Autodesk Inventor part; units mm, degrees
ref_plane "YZ Plane" through (0, 0, 0) normal (1, 0, 0) x (0, 1, 0)
ref_plane "XZ Plane" through (0, 0, 0) normal (0, 1, 0) x (-1, 0, 0)
ref_plane "XY Plane" through (0, 0, 0) normal (0, 0, 1) x (1, 0, 0)
sketch "Sketch1" plane through (0, 0, 0) normal (0, 1, 0) x (-1, 0, 0)
  circle A0 centre (30, -37.5) radius 2
  circle A1 centre (-30, -37.5) radius 2
  circle A2 centre (-30, 37.5) radius 2
  circle A3 centre (30, 37.5) radius 2
  arc A4 (27.9205, -42.0236) -> (32.0065, -32.9436) centre (30, -37.5) ccw
  line L0 (-8.045, -32.9204) -> (0.0364, -32.9204)
  line L1 (-8.045, -32.9204) -> (8.1178, -32.9204)
  line L2 (-8.0814, 33) -> (8.0814, 33)
  line L3 (27.9205, -42.0236) -> (8.1178, -32.9204)
  line L4 (32.0431, -32.9598) -> (8.1178, -22.3088)
  circle A5 centre (-30, -37.5) radius 2
  arc A6 (-31.9701, -32.864) -> (-27.8841, -41.944) centre (-29.9636, -37.4204) ccw
  line L5 (-27.9205, -41.9606) -> (-8.045, -32.9204)
  line L6 (-32.0067, -32.8802) -> (-8.045, -22.213)
  circle A7 centre (30, 37.5) radius 2
  circle A8 centre (-30, 37.5) radius 2
  arc A9 (32.0065, 32.9436) -> (27.9205, 42.0236) centre (30, 37.5) ccw
  line L7 (-8.0814, 33) -> (0, 33)
  line L8 (-8.0814, 33) -> (8.0814, 33)
  line L9 (27.9569, 42.0402) -> (8.0814, 33)
  line L10 (32.0278, 32.953) -> (8.1178, 22.341)
  line L11 (-27.9569, 42.0402) -> (-8.0814, 33)
  circle A10 centre (-30, 37.5) radius 2
  arc A11 (-27.9205, 42.0236) -> (-32.0065, 32.9436) centre (-30, 37.5) ccw
  line L12 (-32.0431, 32.9598) -> (-8.045, 22.2764)
  circle A12 centre (0, -22) radius 1.5
  circle A13 centre (0, 0) radius 1.5
  circle A14 centre (0, 22) radius 1.5
  line L13 (8.1178, 22.341) -> (8.1178, -22.3088)
  line L14 (-8.045, -22.213) -> (-8.045, 22.2764)
extrude "Extrusion1" add sketch "Sketch1" along normal blind 6
sketch "Sketch2" plane through (0, 6, 0) normal (0, 1, 0) x (1, 0, 0)
  circle A0 centre (-30, 37.5) radius 2
  circle A1 centre (-30, 37.5) radius 3.5
  circle A2 centre (30, 37.5) radius 2
  circle A3 centre (30, 37.5) radius 3.5
  circle A4 centre (-30, -37.5) radius 2
  circle A5 centre (-30, -37.5) radius 3.5
  circle A6 centre (30, -37.5) radius 2
  circle A7 centre (30, -37.5) radius 3.5
  point P0 (0, 0)
  dimension "d7" = 7
  dimension "d8" = 7
  dimension "d9" = 7
  dimension "d10" = 7
extrude "Extrusion2" cut sketch "Sketch2" against normal blind 3 contours A1 | A3 | A5 | A6 | A7
sketch "Sketch3" plane through (0, 0, 0) normal (0, -1, 0) x (1, 0, 0)
  circle A0 centre (0, 0) radius 3.5
  circle A1 centre (0, -22) radius 1.5
  circle A2 centre (0, -22) radius 3.5
  circle A3 centre (0, 22) radius 1.5
  circle A4 centre (0, 22) radius 3.5
  dimension "d13" = 7
  dimension "d14" = 7
  dimension "d15" = 7
extrude "Extrusion3" cut sketch "Sketch3" against normal blind 3
properties part number "Battery Plate"
Geometry: final body of the model. Coordinates: model frame, mm. A direction names the side the tool comes from. Coordinates: 2 decimals unless noted, no trailing zeros. Loops run counter-clockwise (first coordinate to the right, second up) from the corner with the lowest first, then second, coordinate; pieces in that order, holes last. Notation, with made-up numbers: M 76,50.5 L 118,50.5 A21 cw 118,88.5 Z; hole C 4.5,56.25 d9. An arc over 180 degrees is marked long. One line per item, written item: value. Start each with the question number.
1) Cut plane C-C (z = -37.5). Return loops of the section in (x, y), then the cut area to 3 significant figures.
2) Draft query along Z for faces 5 (the flat face through (20.175, 2.958, -27.613)), 6 (the flat face through (0, 3, -32.92)), 7 (the flat face through (18.158, 2.958, 37.583)). Return one class per face: released by +Z, released by -Z, zero draft, split by the parting line, or undercut.
3) Pin query (flat end, axial travel): P1, Ø3.5, axis at x = 0, z = -22, coming from the -Y side; P2, Ø5, axis at x = 30, z = 37.5, coming from the -Y side; P3, Ø1.5, axis at x = -7, y = 5.5, coming from the -Z side; P4, Ø1.5, axis at y = 1.5, z = 12, coming from the -X side. Return the tip coordinate at first contact, or that it passes through.
4) Cut plane B-B (x = 20). Return loops of the section in (y, z), then the cut area to 3 significant figures.
5) Cut plane A-A (x = 0). Return loops of the section in (y, z).
6) Material intervals for L1, parallel to Z at x = 0, y = 1.2; L2, parallel to Z at x = 30, y = 1.9; L3, parallel to X at y = 5.05, z = 22 (3 decimals), sorted ascending. Write a range as from..to.
7) Cut plane D-D (y = 4.4). Return loops of the section in (x, z) (1 decimal).
8) Reachability of faces 1 (the flat face through (20.193, 2.958, 27.685)), 2 (the flat face through (-20.229, 2.958, 27.716)), 3 (the cylindrical face through (-0.46, 1.48, -18.53)), 4 (the cylindrical face through (30, 5, -41)) from +Z, -Z, +X, -X, +Y, -Y: full face, straight path, thin tool, end or side. Return the list, or none.
Evaluation:
1. outline: M -34.98,0 L -32,0 L -32,3 L -33.5,3 L -33.5,6 L -34.98,6 Z; M -28,0 L -18.08,0 L -18.08,6 L -26.5,6 L -26.5,3 L -28,3 Z; M 18.11,0 L 28,0 L 28,3 L 26.5,3 L 26.5,6 L 18.11,6 Z; M 32,0 L 34.94,0 L 34.94,6 L 33.5,6 L 33.5,3 L 32,3 Z
1. area: 136 mm^2
2. face 5: undercut
2. face 6: released by -Z
2. face 7: released by +Z
3. P1: y = 3
3. P2: y = 0
3. P3: z = -32.92
3. P4: x = -8.12
4. outline: M 0,-38.36 L 6,-38.36 L 6,-27.54 L 0,-27.54 Z; M 0,27.6 L 6,27.6 L 6,38.42 L 0,38.42 Z
4. area: 130 mm^2
5. outline: M 0,-32.92 L 6,-32.92 L 6,-23.5 L 3,-23.5 L 3,-25.5 L 0,-25.5 Z; M 0,-18.5 L 3,-18.5 L 3,-20.5 L 6,-20.5 L 6,-1.5 L 3,-1.5 L 3,-3.5 L 0,-3.5 Z; M 0,3.5 L 3,3.5 L 3,1.5 L 6,1.5 L 6,20.5 L 3,20.5 L 3,18.5 L 0,18.5 Z; M 0,25.5 L 3,25.5 L 3,23.5 L 6,23.5 L 6,33 L 0,33 Z
6. L1: -32.92..-25.5, -18.5..-3.5, 3.5..18.5, 25.5..33
6. L2: -42.4..-39.5, -35.5..-31.99, 32.05..35.5, 39.5..42.48
6. L3: -8.118..-1.5, 1.5..8.045
7. outline: M -32,-32.9 A5 ccw long -27.9,-42 L -8.1,-32.9 L 8,-32.9 L 27.9,-41.9 A5 ccw long 32,-32.9 L 8,-22.2 L 8,22.3 L 32,32.9 A5 ccw long 28,42 L 8.1,33 L -8.1,33 L -27.9,42 A5 ccw long -32,32.9 L -8.1,22.3 L -8.1,-22.3 Z; hole C -30,-37.5 d7; hole C -30,37.5 d7; hole C 0,-22 d3; hole C 0,0 d3; hole C 0,22 d3; hole C 30,-37.5 d7; hole C 30,37.5 d7
8. face 1: +X, +Y, -Y
8. face 2: -X, +Y, -Y
8. face 3: -Y
8. face 4: +Y
